Autodesk Inventor part; units mm, degrees
ref_plane "YZ Plane" through (0, 0, 0) normal (1, 0, 0) x (0, 1, 0)
ref_plane "XZ Plane" through (0, 0, 0) normal (0, 1, 0) x (-1, 0, 0)
ref_plane "XY Plane" through (0, 0, 0) normal (0, 0, 1) x (1, 0, 0)
sketch "Sketch1" plane through (0, 0, 0) normal (0, 1, 0) x (-1, 0, 0)
  line L0 (0, 0) -> (25.4, 0)
  line L1 (25.4, 0) -> (25.4, -44.45)
  line L2 (25.4, -44.45) -> (0, -44.45)
  line L3 (0, -44.45) -> (0, 0)
  dimension "d0" = 25.4
  dimension "d1" = 44.45
extrude "Extrusion1" add sketch "Sketch1" along normal blind 6.35
fillet "Fillet1" radius 3.048 6 edges at (0, 6.35, -22.225) (0, 0, -22.225) (-12.7, 0, 0) (-12.7, 6.35, 0) (-25.4, 6.35, -22.225) (-25.4, 0, -22.225)
fillet "Fillet2" radius 1.5875 4 edges at (-24.5073, 5.4573, -44.45) (-12.7, 0, -44.45) (-0.8927, 5.4573, -44.45) (-12.7, 6.35, -44.45)
sketch "Sketch2" plane through (-25.4, 3.048, -42.8625) normal (-1, 0, 0) x (0, 0, 1)
  line L0 (0, 0.254) -> (0, 0)
  line L1 (0, 0.127) -> (2.6469, 0.127)
  circle A0 centre (0, 1.3103) radius 0.7937
  circle A1 centre (0, -1.0563) radius 0.7937
  point P0 (42.8625, -3.048)
  dimension "d6" = 1.5875
extrude "Extrusion2" add sketch "Sketch2" along normal mid plane 6.35
properties part number "600mah Battery"
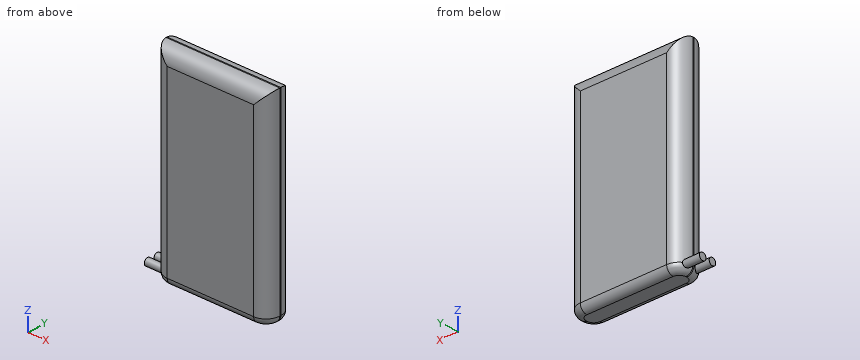
Work out the finished part from the listing and answer in its coordinate system (mm). Round coordinates to 2 decimals unless told otherwise and drop trailing zeros. Order: outer loops, then holes, each group sorted by start corner. A loop starts at its lowest first (then second) coordinate and runs counter-clockwise, first axis right, second up. Notation, with made-up numbers: M 11.5,78.5 L 23.5,78.5 A14 ccw 23.5,88.5 Z; hole C 58,-38 d5. An arc over 180 degrees is marked long. One line per item, written item: value.
Q1. Find section B-B on z = -22. Write down the section's boundary in (x, y).
Derived:
outline: M -25.4,3.05 A3.05 ccw -22.35,0 L -3.05,0 A3.05 ccw 0,3.05 L 0,3.3 A3.05 ccw -3.05,6.35 L -22.35,6.35 A3.05 ccw -25.4,3.3 Z
Q2. A flat-ended cylindrical pin translates along its axis: pin 1 (1.5 mm diameter, centred on y = 2, z = -33.5, fed in from +X). Find the tip coordinate at first contact, or state that the pin passes through.
Derived:
pin 1: x = -0.01
Q3. Straight lines are drawn through the part: line 1 (Z direction, x = -25.75, y = 4.25); line 2 (X direction, y = 3.25, z = -40.5); line 3 (X direction, y = 0.5, z = -33.5). For each, find the intervals that lie inside material, in ascending order.
Derived:
line 1: -43.65 to -42.08
line 2: -25.4 to 0
line 3: -24.02 to -1.38
